Autodesk Fusion 360 part; units mm, degrees
sketch "Sketch1" plane through (0, 0, 0) normal (0, 1, 0) x (1, 0, 0)
  line L0 (0, 0) -> (82, 0)
  line L1 (82, 0) -> (82, -35)
  line L2 (82, -35) -> (0, -35)
  line L3 (0, -35) -> (0, 0)
  line L4 (82, -17.5) -> (69, -17.5) construction
  line L5 (69, -17.5) -> (64.95, -17.5) construction
  line L6 (60.9, -6.45) -> (69, -6.45)
  line L7 (69, -6.45) -> (69, -28.55)
  line L8 (69, -28.55) -> (60.9, -28.55)
  line L9 (60.9, -28.55) -> (60.9, -6.45)
  line L10 (60.9, -6.45) -> (69, -28.55) construction
  line L11 (69, -6.45) -> (60.9, -28.55) construction
  line L12 (82, -35) -> (87, -35)
  line L13 (87, -35) -> (87, 0)
  line L14 (87, 0) -> (82, 0)
  line L15 (82, 0) -> (82, -35)
  line L16 (0, -35) -> (-5, -35)
  line L17 (-5, -35) -> (-5, 0)
  line L18 (-5, 0) -> (0, 0)
  line L19 (0, 0) -> (0, -35)
  line L20 (71.95, -20) -> (57.95, -20)
  line L21 (57.95, -20) -> (57.95, -15)
  line L22 (57.95, -15) -> (71.95, -15)
  line L23 (71.95, -15) -> (71.95, -20)
  line L24 (71.95, -20) -> (57.95, -15) construction
  line L25 (57.95, -20) -> (71.95, -15) construction
  point P0 (64.95, -17.5)
  point P1 (64.95, -17.5)
  dimension "d1" = 82
  dimension "d2" = 35
  dimension "d3" = 13
  dimension "d4" = 4.05
  dimension "d5" = 8.1
  dimension "d6" = 22.1
  dimension "d7" = 5
  dimension "d8" = 35
  dimension "d9" = 5
  dimension "d10" = 35
  dimension "d15" = 14
  dimension "d16" = 5
extrude "Extrude1" add sketch "Sketch1" along normal blind 15 contours L3 L16 L17 L18 L19 | L1 L12 L13 L14 L15 makes body 1 at (0, 5, 23.3333) makes body 2 at (87, 5, 23.3333)
extrude "Extrude2" add sketch "Sketch1" along normal blind 4 contours L0 L1 L2 L3 L15 L19 | L9 L20 L21 L22 | L7 L20 L22 L23 bodies 1 2
extrude "Extrude3" cut sketch "Sketch1" along normal blind 4 contours L9 L20 L21 L22 | L7 L20 L22 L23 bodies 1
equation "d4 = ( 8.1 / 2 ) * 1 mm"
Here's how the part is built. I have some questions about the finished solid (model axes, mm). A direction names the side the tool comes from. Coordinates: 2 decimals unless noted, no trailing zeros. Order: outer loops, then holes, each group sorted by start corner. A loop starts at its lowest first (then second) coordinate and runs counter-clockwise, first axis right, second up. Notation, with made-up numbers: M 34,-24.5 L 63,-24.5 A22 ccw 63,-12.5 Z; hole C 46.25,34 d9. An arc over 180 degrees is marked long. Answer as CSV lines item,"result". Start each with the question number.
1. I need wall thicknesses on line 1 (X direction, y = 4.75, z = 3); line 2 (Y direction, x = 69, z = 6); line 3 (X direction, y = 1.75, z = 28). Which ranges of each line are inside material? Lowest first, please. Write a range as [from, to].
2. I want a section at A-A, the plane x = 65.5. Write out the boundary of the cut face in (y, z), and give its area (3 significant figures).
3. I want a section at D-D, the plane z = 5.5. Write out the boundary of the cut face in (x, y), and give its area (3 significant figures).
4. On a 3-axis mill with a long thin cutter (end or side, diameter ignored), from which of +Z, -Z, +X, -X, +Y, -Y can I reach the whole of each face in a straight line? I mean faces 5 (the flat face through (40, 0, 17)), 6 (the flat face through (69, 2, 24)), 7 (the flat face through (40, 4, 17)). Say none if no direction works.
5. I want a section at C-C, the plane z = 25.5. Write out the boundary of the cut face in (x, y), and give its area (3 significant figures).
6. I want a section at B-B, the plane y = 10.5. Write out the boundary of the cut face in (x, z).
7. For pin 1 (5 mm diameter, centred on x = 66, z = 8.5, fed in from +Y), with a flat end and sliding along its axis, tell me the tip position at first contact or that it passes through.
8. We'd pull the mould along Z, two halves only. Please class faces 1 (the flat face through (82, 9, 17)), 2 (the flat face through (59, 2, 20)), 3 (the flat face through (37, 3, 0)), 4 (the flat face through (71.95, 2, 17)): released by +Z, released by -Z, zero draft, split by the parting line, or undercut.
Recorded:
1,line 1,"x = [-5, 0], [82, 87]"
1,line 2,"y = [0, 4]"
1,line 3,"x = [-5, 60.9], [69, 87]"
2,outline,"M 0,0 L 4,0 L 4,6.45 L 0,6.45 Z; M 0,28.55 L 4,28.55 L 4,35 L 0,35 Z"
2,area,"51.6 mm2"
3,outline,"M -5,0 L 87,0 L 87,15 L 82,15 L 82,4 L 0,4 L 0,15 L -5,15 Z"
3,area,"478 mm2"
4,face 5,"+Z, -Z, +X, -X, -Y"
4,face 6,"+Y, -Y"
4,face 7,"+Z, -Z, +Y"
5,outline,"M -5,0 L 60.9,0 L 60.9,4 L 0,4 L 0,15 L -5,15 Z; M 69,0 L 87,0 L 87,15 L 82,15 L 82,4 L 69,4 Z"
5,area,"446 mm2"
6,outline,"M -5,0 L 0,0 L 0,35 L -5,35 Z; M 82,0 L 87,0 L 87,35 L 82,35 Z"
7,pin 1,"stops at y = 4"
8,face 1,"zero draft"
8,face 2,"undercut"
8,face 3,"released by -Z"
8,face 4,"undercut"
